Design review of the part built by this model. Coordinates are the model's own, in mm. A direction names the side the tool comes from. Coordinates: 2 decimals unless noted, no trailing zeros. Loops run counter-clockwise (first coordinate to the right, second up) from the corner with the lowest first, then second, coordinate; pieces in that order, holes last. Notation, with made-up numbers: (78, 6) -> (136, 6) arc R28 cw to (136, 33) -> close; hole circle Ø11 at (61.5, 66.25). An arc over 180 degrees is marked (long way). One line per item, written item: value. Start each with the question number.
1. Insertion check: pin 1 (10 mm diameter, centred on x = 2, y = 15, fed in from +Z); pin 2 (3 mm diameter, centred on x = -7, z = 9.5, fed in from -Y); pin 3 (3 mm diameter, centred on x = 0, y = -13.9, fed in from -Z). Each pin has a flat end and moves straight along its axis. Give the tip position at first contact, or say it passes through.
2. Add section A-A on z = 2.75. Write out the cut boundary in (x, y), plus the area to 3 significant figures.
3. Add section B-B on y = -13.9. Write out the cut boundary in (x, z).
4. Add section D-D on y = -5.5. Write out the cut boundary in (x, z), plus the area to 3 significant figures.
5. Draft analysis for pull direction X (two halves, no side actions). For faces 1 (the cylindrical face through (-4, 18, 3)), 2 (the cylindrical face through (0.13, -14.89, 2.54)), 3 (the flat face through (7, 0, 2)), 4 (the flat face through (-7, 47, 3)), state which applies: pulls with the +X half, pulls with the -X half, needs draft (parallel to the pull), parting line crosses it, or undercut.
6. For probe 1 along Y at (x, z) = (-6, 2.5); probe 2 along X at (y, z) = (-13.9, 1); probe 3 along Y at (x, z) = (0, 1.6), list the stretches that pass through material, from the lowest coordinate up.
7. Add section C-C on x = 0. Write out the cut boundary in (y, z).
8. Machinability: for faces 5 (the cylindrical face through (-7.465, 51.787, 11.748)), 6 (the flat face through (-8, 17.5, -4)), 7 (the flat face through (-7, 35, -4.5)), 8 (the cylindrical face through (-9, -17, 3)), 9 (the flat face through (-7, 0, 2)), which of the approach directions +Z, -Z, +X, -X, +Y, -Y give a long, thin tool a straight path to every point of the face, cutting with its end or side? Answer none if there is none.
```python
from build123d import *

# Parameters (mm, degrees)
SKETCH1_W           = 20
SKETCH1_H           = 35
SKETCH1_W_2         = 14
SKETCH1_H_2         = 24
BOSS_EXTRUDE1_DEPTH = 5
SKETCH2_R           = 1
CUT_EXTRUDE1_DEPTH  = 5
BOSS_EXTRUDE2_DEPTH = 5
FILLET1_R           = 2.5
FILLET2_R           = 2.5
SKETCH5_R           = 1
SKETCH5_W           = 14
SKETCH5_H           = 24
CUT_EXTRUDE2_DEPTH  = 10


with BuildPart() as part:
    # Sketch1 → Boss-Extrude1 (new body)
    with BuildSketch(Plane.XY):
        Rectangle(SKETCH1_W, SKETCH1_H)
        Rectangle(SKETCH1_W_2, SKETCH1_H_2, mode=Mode.SUBTRACT)
    extrude(amount=BOSS_EXTRUDE1_DEPTH)

    # Sketch2 → Cut-Extrude1 (cut)
    with BuildSketch(Plane.XY.offset(5)):
        with Locations((0, 13.9)):
            Circle(SKETCH2_R)
        with Locations(Location((0, -13.9, 0), (0, 0, 180))):
            Circle(SKETCH2_R)
    extrude(amount=-CUT_EXTRUDE1_DEPTH, mode=Mode.SUBTRACT)

    # Sketch3 → Boss-Extrude2 (add)
    with BuildSketch(Plane.ZY.offset(10)):
        Polygon((-7.5, 52.5), (-7.5, 17.5), (0, 17.5), (2.5, 17.5), (2.5, 52.5), align=None)
        Polygon((2.5, 52.5), (2.5, 17.5), (5, 17.5), (12.5, 17.5), (12.5, 52.5), align=None)
    extrude(amount=-BOSS_EXTRUDE2_DEPTH)

    # Fillet1
    fillet1_edges = [part.edges().sort_by_distance(p)[0] for p in [
        (-7.5, 17.5, 0),
        (-7.5, 17.5, 5),
    ]]
    fillet(fillet1_edges, radius=FILLET1_R)

    # Fillet2
    fillet2_edges = [part.edges().sort_by_distance(p)[0] for p in [
        (-5, 17.5, 2.5),
        (-7.5, 17.5, 12.5),
        (-7.5, 17.5, -7.5),
        (-7.5, 52.5, -7.5),
        (-7.5, 52.5, 12.5),
        (10, -17.5, 2.5),
        (-10, -17.5, 2.5),
        (10, 17.5, 2.5),
    ]]
    fillet(fillet2_edges, radius=FILLET2_R)

    # Sketch5 → Cut-Extrude2 (cut)
    with BuildSketch(Plane(origin=(-5, 0, 0), x_dir=(0, 0, -1), z_dir=(1, 0, 0))):
        with Locations((-2.5, 21.1)):
            Circle(SKETCH5_R)
        with Locations((-2.5, 48.9)):
            Circle(SKETCH5_R)
        with Locations((-2.5, 35)):
            Rectangle(SKETCH5_W, SKETCH5_H)
    extrude(amount=-CUT_EXTRUDE2_DEPTH, mode=Mode.SUBTRACT)


solid = part.part
```
Worked answers:
1. pin 1: stops at z = 5
1. pin 2: stops at y = 17.5
1. pin 3: stops at z = 0
2. outline: (-10, -15) arc R2.5 ccw to (-7.5, -17.5) -> (7.5, -17.5) arc R2.5 ccw to (10, -15) -> (10, 15) arc R2.5 ccw to (7.5, 17.5) -> (-2.5, 17.5) arc R2.5 cw to (-5, 20) -> (-5, 20.13) -> (-10, 20.13) -> close; (-10, 22.07) -> (-5, 22.07) -> (-5, 23) -> (-10, 23) -> close; (-10, 47) -> (-5, 47) -> (-5, 47.93) -> (-10, 47.93) -> close; (-10, 49.87) -> (-5, 49.87) -> (-5, 52.5) -> (-10, 52.5) -> close; hole (-7, -12) -> (7, -12) -> (7, 12) -> (-7, 12) -> close; hole circle Ø2 at (0, -13.9); hole circle Ø2 at (0, 13.9)
2. area: 391 mm²
3. outline: (-10, 0) -> (-1, 0) -> (-1, 5) -> (-10, 5) -> close; (1, 0) -> (10, 0) -> (10, 5) -> (1, 5) -> close
4. outline: (-10, 0) -> (-7, 0) -> (-7, 5) -> (-10, 5) -> close; (7, 0) -> (10, 0) -> (10, 5) -> (7, 5) -> close
4. area: 30.0 mm²
5. face 1: pulls with the +X half
5. face 2: undercut
5. face 3: undercut
5. face 4: needs draft
6. probe 1: y = -17.5 to -12, 12 to 20.1, 22.1 to 23, 47 to 47.9, 49.9 to 52.5
6. probe 2: x = -10 to -1, 1 to 10
6. probe 3: y = -17.5 to -14.9, -12.9 to -12, 12 to 12.9, 14.9 to 17.5
7. outline: (-17.5, 0) -> (-14.9, 0) -> (-14.9, 5) -> (-17.5, 5) -> close; (-12.9, 0) -> (-12, 0) -> (-12, 5) -> (-12.9, 5) -> close; (12, 0) -> (12.9, 0) -> (12.9, 5) -> (12, 5) -> close; (14.9, 0) -> (17.5, 0) -> (17.5, 5) -> (14.9, 5) -> close
8. face 5: +Z, +X, -X, +Y
8. face 6: -Z, +X, -X, -Y
8. face 7: +X, -X
8. face 8: +Z, -Z, -X, -Y
8. face 9: +Z, -Z
